CAD build for the part. Positions are in the model's coordinates, mm. Face numbers are marked on the shaded views. A direction names the side the tool comes from. Give positions to 0.01 mm unless a question says otherwise; leave off trailing zeros. Loops run counter-clockwise (first coordinate to the right, second up) from the corner with the lowest first, then second, coordinate; pieces in that order, holes last. Notation, with made-up numbers: (31.25, 88.5) - (59.25, 88.5) arc R35 ccw to (59.25, 120.5) - close; hole circle Ø10 at (-28.75, 39.5). An arc over 180 degrees is marked (long way). Return JSON: item names as keys, results as strings.
from build123d import *

# Parameters (mm, degrees)
CUT_EXTRUDE_1_DEPTH = 23.181073013
CHAMFER_1_SIZE      = 0.25
HOLE_WIZARD_1_D     = 3.5


# Read off the part's stored shape, not the designer's step: M3 螺纹孔3
with BuildPart() as part:
    # 草图2 → 旋转1 (revolve)
    with BuildSketch(Plane.XY, mode=Mode.PRIVATE) as revolve_1_sk:
        Polygon((18, 4), (18, 6), (10, 6), (10, 14), (5, 14), (5, 5.75), (4.5, 5.75), (4.5, 6), (0, 6), (0, 4), align=None)
    revolve(revolve_1_sk.sketch.rotate(Axis((0, 0, 0), (1, 0, 0)), 90), axis=Axis((0, 0, 0), (1, 0, 0)))

    # 草图3 → 切除-拉伸1 (cut, through all)
    with BuildSketch(Plane(origin=(10, 0, 0), x_dir=(0, 0, -1), z_dir=(1, 0, 0))):
        with BuildLine():
            Line((-8, -11.489125293), (-8, 11.489125293))
            ThreePointArc((-8, 11.489125293), (-14, 0), (-8, -11.489125293))
        make_face()
        with BuildLine():
            ThreePointArc((14, 0), (12.409673646, 6.480740698), (8, 11.489125293))
            Line((8, 11.489125293), (8, -11.489125293))
            ThreePointArc((8, -11.489125293), (12.409673646, -6.480740698), (14, 0))
        make_face()
    extrude(amount=-CUT_EXTRUDE_1_DEPTH, mode=Mode.SUBTRACT)

    # 倒角1
    chamfer_1_edges = [part.edges().sort_by_distance(p)[0] for p in [
        (0, 0, -6),
    ]]
    chamfer(chamfer_1_edges, length=CHAMFER_1_SIZE)

    # 孔1 (through all)
    with Locations(Plane(origin=(10, 0, 0), x_dir=(0, 0, -1), z_dir=(1, 0, 0))):
        with Locations((0, 10), (0, -10)):
            Hole(HOLE_WIZARD_1_D / 2)

    # M3 螺纹孔3 outline → M3 螺纹孔3 (revolve, cut)
    with BuildSketch(Plane(origin=(14, 0, 0), x_dir=(1, 0, 0), z_dir=(0, 0.707106781186545, 0.70710678118655))):
        Polygon((1.525087405, 6.000087405), (0, 6.000087405), (0, 3.799554737), (1.25, 3.799554737), (1.25, 5.725), align=None)
    revolve(axis=Axis((14, 0, 0), (0, 0.70710678118655, -0.707106781186545)), mode=Mode.SUBTRACT)

    # Hole Wizard M3 _3 2 outline → Hole Wizard M3 _3 2 (revolve, cut)
    with BuildSketch(Plane(origin=(14, 0, 0), x_dir=(1, 0, 0), z_dir=(0, -0.707106781186542, 0.707106781186553))):
        Polygon((0, -6.000094082), (1.525094082, -6.000094082), (1.25, -5.725), (1.25, -3.799554737), (0, -3.799554737), align=None)
    revolve(axis=Axis((14, 0, 0), (0, 0.707106781186553, 0.707106781186542)), mode=Mode.SUBTRACT)


solid = part.part
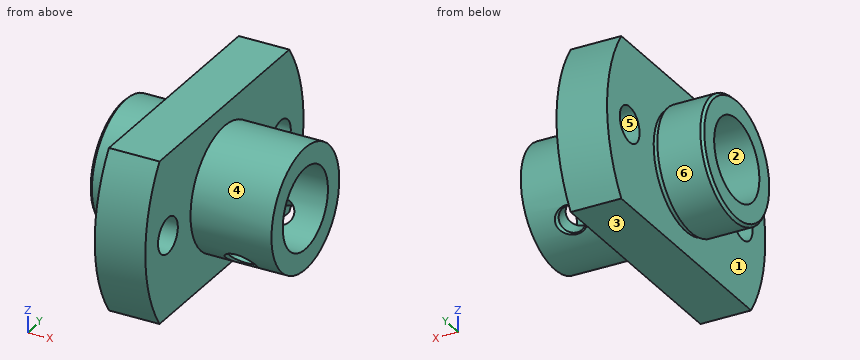
1. Cut at B-B, the plane z = 0. Give the number of separate pieces and of enclosed holes in the cut face, plus the area to 3 significant figures.
Values follow:
{"separate pieces": "4", "enclosed holes": "0", "area": "117 mm²"}
2. Cut at C-C, the plane x = 8. Write the cut outline in (y, z).
Values follow:
{"outline": "(-11.49, -8) - (11.49, -8) arc R14 ccw to (11.49, 8) - (-11.49, 8) arc R14 ccw to start; hole circle Ø3.5 at (-10, 0); hole circle Ø8 at (0, 0); hole circle Ø3.5 at (10, 0)"}
3. Drill centre lines: probe 1 along Y at (x, z) = (11.25, 0.25); probe 2 along Y at (x, z) = (6.25, -1.5); probe 3 along X at (y, z) = (11.5, 5.75). Where is each one in solid material? Low to high.
Values follow:
{"probe 1": "y = -5.99 to -3.99, 3.99 to 5.99", "probe 2": "y = -13.92 to -10.9, -9.1 to -3.71, 3.71 to 9.1, 10.9 to 13.92", "probe 3": "x = 5 to 10"}
4. Cut at D-D, the plane x = 1.75. Write the cut outline in (y, z), plus the area to 3 significant figures.
Values follow:
{"outline": "circle Ø12 at (0, 0); hole circle Ø8 at (0, 0)", "area": "62.8 mm²"}
5. Drop flat-ended pins along their axis: P1, Ø3, axis at y = -10, z = 5, coming from the +X side; P2, Ø1.5, axis at x = 2, z = -4.5, coming from the -Y side; P3, Ø1.5, axis at x = 4, y = 1, coming from the -Z side; P4, Ø3, axis at y = 10, z = 0, coming from the -X side. Give the stop position or say it passes through.
Values follow:
{"P1": "stops at x = 10", "P2": "stops at y = -4.68", "P3": "stops at z = -5.99", "P4": "passes through"}
6. Pull direction Z, two halves, no side cores. Call the marked faces 1, 2 and 3: +Z half, -Z half, draft (parallel to the pull), parting line (faces both ways), or undercut.
Values follow:
{"face 1": "draft", "face 2": "undercut", "face 3": "-Z half"}
7. Which spindle directions (+Z, -Z, +X, -X, +Y, -Y) get a long thin tool onto all of the face, cutting with end or side? Do the marked faces 4, 5 and 6. Say none if no direction does.
Values follow:
{"face 4": "+X", "face 5": "+X, -X", "face 6": "-X"}
8. Cut at A-A, the plane y = 10. Write the cut outline in (x, z), plus the area to 3 significant figures.
Values follow:
{"outline": "(5, -8) - (10, -8) - (10, -1.75) - (5, -1.75) - close; (5, 1.75) - (10, 1.75) - (10, 8) - (5, 8) - close", "area": "62.5 mm²"}
